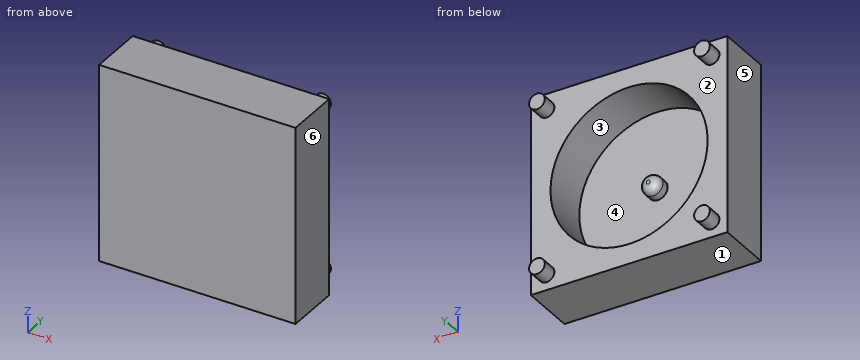
```python
from build123d import *

# Parameters (mm, degrees)
SKETCH1_W           = 25
SKETCH1_H           = 25
BOSS_EXTRUDE1_DEPTH = 7
SKETCH2_R           = 10
CUT_EXTRUDE1_DEPTH  = 6
SKETCH3_R           = 1.25
BOSS_EXTRUDE2_DEPTH = 2
FILLET1_R           = 1
SKETCH4_R           = 1
BOSS_EXTRUDE3_DEPTH = 2


with BuildPart() as part:
    # Sketch1 → Boss-Extrude1 (new body)
    with BuildSketch(Plane(origin=(0, 0, 0), x_dir=(1, 0, 0), z_dir=(0, 1, 0))):
        Rectangle(SKETCH1_W, SKETCH1_H)
    extrude(amount=BOSS_EXTRUDE1_DEPTH)

    # Sketch2 → Cut-Extrude1 (cut)
    with BuildSketch(Plane(origin=(0, 7, 0), x_dir=(1, 0, 0), z_dir=(0, 1, 0))):
        Circle(SKETCH2_R)
    extrude(amount=-CUT_EXTRUDE1_DEPTH, mode=Mode.SUBTRACT)

    # Sketch3 → Boss-Extrude2 (add)
    with BuildSketch(Plane(origin=(0, 1, 0), x_dir=(1, 0, 0), z_dir=(0, 1, 0))):
        Circle(SKETCH3_R)
    extrude(amount=BOSS_EXTRUDE2_DEPTH)

    # Fillet1
    fillet1_edges = [part.edges().sort_by_distance(p)[0] for p in [
        (-1.25, 3, 0),
    ]]
    fillet(fillet1_edges, radius=FILLET1_R)

    # Sketch4 → Boss-Extrude3 (add)
    with BuildSketch(Plane(origin=(0, 7, 0), x_dir=(1, 0, 0), z_dir=(0, 1, 0))):
        with Locations((-10.5, 10.5)):
            Circle(SKETCH4_R)
        with Locations((10.5, 10.5)):
            Circle(SKETCH4_R)
        with Locations((10.5, -10.5)):
            Circle(SKETCH4_R)
        with Locations((-10.5, -10.5)):
            Circle(SKETCH4_R)
    extrude(amount=BOSS_EXTRUDE3_DEPTH)


solid = part.part
```
Geometry check sheet. Reference: the model listing, model coordinates, mm. Face numbers are marked on the shaded views. A direction names the side the tool comes from. Round coordinates to 2 decimals unless told otherwise and drop trailing zeros. Loops run counter-clockwise (first coordinate to the right, second up) from the corner with the lowest first, then second, coordinate; pieces in that order, holes last. Notation, with made-up numbers: (60, 44.5) -> (111, 44.5) arc R14 cw to (111, 56.5) -> close; hole circle Ø5 at (-7, 20). An arc over 180 degrees is marked (long way). Use a Markdown table: item, result.
(1) Sectioned sample at D-D (z = -6). Enter the section's corners in (x, y), then the cut area to 3 significant figures.
Calculated:
| item | result |
|---|---|
| outline | (-12.5, 0) -> (12.5, 0) -> (12.5, 7) -> (8, 7) -> (8, 1) -> (-8, 1) -> (-8, 7) -> (-12.5, 7) -> close |
| area | 79.0 mm² |
(2) Scan lines: probe 1 along Z at (x, y) = (0, 4.35); probe 2 along X at (y, z) = (2.45, 0). Record each from-to range of solid material in increasing order.
Calculated:
| item | result |
|---|---|
| probe 1 | -12.5 to -10, 10 to 12.5 |
| probe 2 | -12.5 to -10, -1.14 to 1.14, 10 to 12.5 |
(3) Sectioned sample at C-C (z = -10.5). Enter the section's corners in (x, y), then the cut area to 3 significant figures.
Calculated:
| item | result |
|---|---|
| outline | (-12.5, 0) -> (12.5, 0) -> (12.5, 7) -> (11.5, 7) -> (11.5, 9) -> (9.5, 9) -> (9.5, 7) -> (-9.5, 7) -> (-9.5, 9) -> (-11.5, 9) -> (-11.5, 7) -> (-12.5, 7) -> close |
| area | 183 mm² |
(4) Set-up check for the marked faces 1 and 2: record each of +Z, -Z, +X, -X, +Y, -Y from which the full face is reachable in a straight line by a thin tool's end or side.
Calculated:
| item | result |
|---|---|
| face 1 | -Z, +X, -X, +Y, -Y |
| face 2 | +Y |
(5) Sectioned sample at A-A (x = -10.5). Enter the section's corners in (y, z).
Calculated:
| item | result |
|---|---|
| outline | (0, -12.5) -> (7, -12.5) -> (7, -11.5) -> (9, -11.5) -> (9, -9.5) -> (7, -9.5) -> (7, 9.5) -> (9, 9.5) -> (9, 11.5) -> (7, 11.5) -> (7, 12.5) -> (0, 12.5) -> close |
(6) Sectioned sample at B-B (y = 3.75). Enter the section's corners in (x, z).
Calculated:
| item | result |
|---|---|
| outline | (-12.5, -12.5) -> (12.5, -12.5) -> (12.5, 12.5) -> (-12.5, 12.5) -> close; hole circle Ø20 at (0, 0) |
(7) Mould release check, pull along X, two halves, no side actions. Record for the marked faces 3, 4, 5 and 6: released by +X, released by -X, zero draft, split by the parting line, or undercut.
Calculated:
| item | result |
|---|---|
| face 3 | undercut |
| face 4 | undercut |
| face 5 | released by -X |
| face 6 | released by +X |
(8) Go/stop test with flat-tipped pins: P1, Ø1, axis at x = -3, z = -2.5, coming from the +Y side; P2, Ø4, axis at x = 9, z = -3.5, coming from the +Y side; P3, Ø7.5, axis at x = 3, z = -0.5, coming from the +Y side. Record where each tip stops, or that it passes through.
Calculated:
| item | result |
|---|---|
| P1 | y = 1 |
| P2 | y = 7 |
| P3 | y = 3 |
